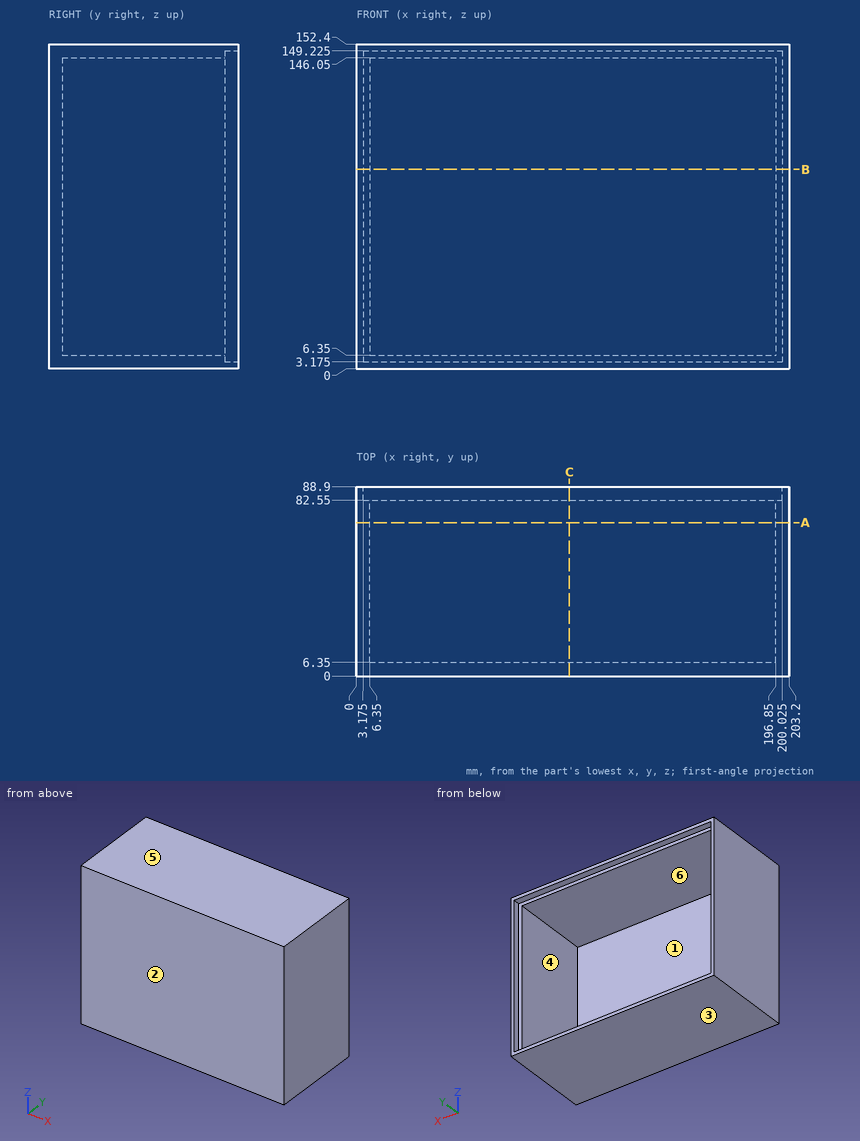
Geometry check sheet. Reference: drawing and pictorial views, mm from the part's lowest x, y, z. A direction names the side the tool comes from. Give positions to 0.01 mm unless a question says otherwise; leave off trailing zeros. Order: outer loops, then holes, each group sorted by start corner. A loop starts at its lowest first (then second) coordinate and runs counter-clockwise, first axis right, second up. Notation, with made-up numbers: M -9.5,-22 L 17.5,-22 A27 ccw 17.5,-4 Z; hole C 54.5,87 d8. An arc over 180 degrees is marked long. Answer in a Markdown table with one row per item. Add a question column.
Q1. Sectioned sample at A-A, the plane y = 72. Record the boundary of the cut face in (x, z).
Q2. Access from +Z, -Z, +X, -X, +Y, -Y to the whole of each face (thin tool, end or side, straight path). Record for the marked faces 5 and 6.
Q3. Sectioned sample at B-B, the plane z = 93.5. Record the boundary of the cut face in (x, y) (3 decimals).
Q4. Sectioned sample at C-C, the plane x = 100. Record the boundary of the cut face in (y, z) (3 decimals), and give its area (3 significant figures).
Q5. Release check for a two-part mould opening along Z. For the marked faces 1, 2, 3 and 4 record: released by +Z, released by -Z, zero draft, split by the parting line, or undercut.
Q6. Thickness scan on L1, parallel to Z at x = 66.5, y = 30.5; L2, parallel to X at y = 10, z = 26.5; L3, parallel to Y at x = 173.5, z = 118.5. Record the ranges inside material, lowest first.
Q7. Gauge pin test, flat ends, axial feed: pin 1 Ø5 at (y, z) = (51, 127.5) entering from -X; pin 2 Ø2 at (x, z) = (72.5, 127.5) entering from +Y. Record the tip position at first contact, or that the pin passes through.
Verdict:
| question | item | result |
|---|---|---|
| 1 | outline | M 0,0 L 203.2,0 L 203.2,152.4 L 0,152.4 Z; hole M 6.35,6.35 L 196.85,6.35 L 196.85,146.05 L 6.35,146.05 Z |
| 2 | face 5 | +Z, +X, -X, +Y, -Y |
| 2 | face 6 | +Y |
| 3 | outline | M 0,0 L 203.2,0 L 203.2,88.9 L 200.025,88.9 L 200.025,82.55 L 196.85,82.55 L 196.85,6.35 L 6.35,6.35 L 6.35,82.55 L 3.175,82.55 L 3.175,88.9 L 0,88.9 Z |
| 4 | outline | M 0,0 L 88.9,0 L 88.9,3.175 L 82.55,3.175 L 82.55,6.35 L 6.35,6.35 L 6.35,146.05 L 82.55,146.05 L 82.55,149.225 L 88.9,149.225 L 88.9,152.4 L 0,152.4 Z |
| 4 | area | 1,980 mm² |
| 5 | face 1 | undercut |
| 5 | face 2 | zero draft |
| 5 | face 3 | released by -Z |
| 5 | face 4 | undercut |
| 6 | L1 | 0 to 6.35, 146.05 to 152.4 |
| 6 | L2 | 0 to 6.35, 196.85 to 203.2 |
| 6 | L3 | 0 to 6.35 |
| 7 | pin 1 | x = 0 |
| 7 | pin 2 | y = 6.35 |
